```python
from build123d import *

# Parameters (mm, degrees)
PAD001_DEPTH = 8.4
SKETCH001_W  = 7
SKETCH001_H  = 10.8
PAD_DEPTH    = 3


with BuildPart() as part:
    # Sketch → Pad001 (new body)
    with BuildSketch(Plane.XZ):
        Polygon((0, 0), (0, 10.8), (4.4, 10.8), (4.4, 3.1), (7.5, 3.1), (7.5, 10.8), (11.9, 10.8), (11.9, 0), align=None)
    extrude(amount=-PAD001_DEPTH)

    # Sketch001 → Pad (join)
    with BuildSketch(Plane.XZ):
        with Locations((-3.5, 5.4)):
            Rectangle(SKETCH001_W, SKETCH001_H)
    extrude(amount=-PAD_DEPTH)


solid = part.part
```
Model file for the job. Use its own axes, mm. A direction names the side the tool comes from. Coordinates: 2 decimals unless noted, no trailing zeros. Write each loop counter-clockwise with the first axis right and the second up, starting at its lowest first coordinate (ties: lowest second). Pieces come first, ordered by that corner, then holes. Notation, with made-up numbers: (24, -37.75) - (67, -37.75) arc R27 ccw to (67, -5.75) - close; hole circle Ø11 at (52.5, 58). An arc over 180 degrees is marked (long way). Use a Markdown table: item, result. Add a question column.
Item 1: Drop flat-ended pins along their axis: pin 1 (2.5 mm diameter, centred on y = 5.5, z = 4, fed in from -X); pin 2 (1.5 mm diameter, centred on x = 5.5, y = 5.5, fed in from +Z). Give the stop position or say it passes through.
Item 2: Band-saw the part on A-A, the plane z = 5.5. Write the cut outline in (x, y).
Item 3: 3-axis set-ups, long thin cutter, end or side, ignore diameter. For faces 4 (the face through (-4, 3, 5)), 5 (the face through (2, 0, 5)), 6 (the face through (7.5, 4, 7)): which of +Z, -Z, +X, -X, +Y, -Y reach the whole face in a straight line?
Item 4: Band-saw the part on C-C, the plane z = 2.25. Write the cut outline in (x, y).
Item 5: Drill centre lines: line 1 along X through (y, z) = (1, 9.75); line 2 along X through (y, z) = (5.25, 5.75); line 3 along Y through (x, z) = (-5, 7.75). Where is each one in solid material? Low to high.
Item 6: Two-plate mould, pull along X, no slides. Class faces 1 (the face through (4.4, 4, 7)), 2 (the face through (0, 6, 5)), 3 (the face through (0, 2, 10.8)): pulls with the +X half, pulls with the -X half, needs draft (parallel to the pull), parting line crosses it, or undercut.
Item 7: Band-saw the part on D-D, the plane x = -1. Write the cut outline in (y, z), and give its area (3 significant figures).
Item 8: Band-saw the part on B-B, the plane y = 6.75. Write the cut outline in (x, z), and give its area (3 significant figures).
A:
| question | item | result |
|---|---|---|
| 1 | pin 1 | stops at x = 0 |
| 1 | pin 2 | stops at z = 3.1 |
| 2 | outline | (-7, 0) - (4.4, 0) - (4.4, 8.4) - (0, 8.4) - (0, 3) - (-7, 3) - close; (7.5, 0) - (11.9, 0) - (11.9, 8.4) - (7.5, 8.4) - close |
| 3 | face 4 | +Z, -Z, -X, +Y |
| 3 | face 5 | +Z, -Z, +X, -X, -Y |
| 3 | face 6 | +Z, +Y, -Y |
| 4 | outline | (-7, 0) - (11.9, 0) - (11.9, 8.4) - (0, 8.4) - (0, 3) - (-7, 3) - close |
| 5 | line 1 | x = -7 to 4.4, 7.5 to 11.9 |
| 5 | line 2 | x = 0 to 4.4, 7.5 to 11.9 |
| 5 | line 3 | y = 0 to 3 |
| 6 | face 1 | undercut |
| 6 | face 2 | pulls with the -X half |
| 6 | face 3 | needs draft |
| 7 | outline | (0, 0) - (3, 0) - (3, 10.8) - (0, 10.8) - close |
| 7 | area | 32.4 mm² |
| 8 | outline | (0, 0) - (11.9, 0) - (11.9, 10.8) - (7.5, 10.8) - (7.5, 3.1) - (4.4, 3.1) - (4.4, 10.8) - (0, 10.8) - close |
| 8 | area | 105 mm² |
